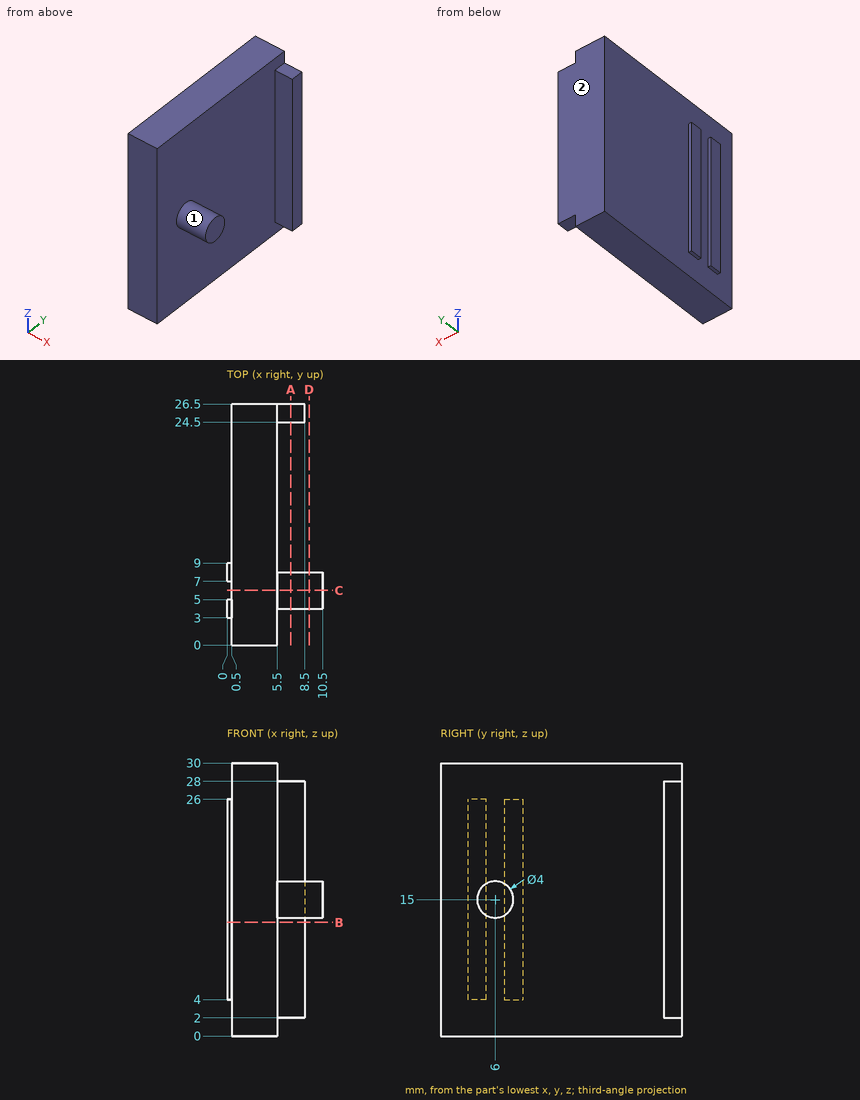
Geometry: see drawing. Coordinates: mm, zero at the bounding-box minimum. A direction names the side the tool comes from. Coordinates: 2 decimals unless noted, no trailing zeros. Loops run counter-clockwise (first coordinate to the right, second up) from the corner with the lowest first, then second, coordinate; pieces in that order, holes last. Notation, with made-up numbers: M -5,-26 L 12,-26 A18 ccw 12,-15 Z; hole C 73,-36 d8. An arc over 180 degrees is marked long. Put each result on its own line as item: value. Start each with the question number.
1) Contact query for flat-ended pins moving along their axis: pin 1 Ø3 at (y, z) = (6, 8) entering from +X; pin 2 Ø8 at (y, z) = (14.5, 12.5) entering from -X; pin 3 Ø0.6 at (y, z) = (25.5, 15) entering from +X. Output: stop coordinate, or through.
2) Cut plane D-D on x = 9. Return the cut outline in (y, z), then the cut area to 3 significant figures.
3) Ray query, L1, parallel to X at y = 20, z = 19.75; L2, parallel to X at y = 7.25, z = 8; L3, parallel to Y at x = 7.25, z = 8.5. Return the intervals inside material, ascending. Write a range as from..to.
4) Cut plane A-A on x = 7. Return the cut outline in (y, z), then the cut area to 3 significant figures.
5) Reachability of the marked faces 1 and 2 from +Z, -Z, +X, -X, +Y, -Y: full face, straight path, thin tool, end or side. Return the list, or none.
6) Cut plane B-B on z = 12.5. Return the cut outline in (x, y), then the cut area to 4 significant figures.
7) Cut plane C-C on y = 6. Return the cut outline in (x, z), then the cut area to 3 significant figures.
The answers:
1. pin 1: stops at x = 5.5
1. pin 2: stops at x = 0.5
1. pin 3: stops at x = 8.5
2. outline: C 6,15 d4
2. area: 12.6 mm²
3. L1: x = 0.5..5.5
3. L2: x = 0..5.5
3. L3: y = 24.5..26.5
4. outline: C 6,15 d4; M 24.5,2 L 26.5,2 L 26.5,28 L 24.5,28 Z
4. area: 64.6 mm²
5. face 1: +X
5. face 2: +Z, -Z, +X, -X, +Y
6. outline: M 0,3 L 0.5,3 L 0.5,0 L 5.5,0 L 5.5,24.5 L 8.5,24.5 L 8.5,26.5 L 0.5,26.5 L 0.5,9 L 0,9 L 0,7 L 0.5,7 L 0.5,5 L 0,5 Z
6. area: 140.5 mm²
7. outline: M 0.5,0 L 5.5,0 L 5.5,13 L 10.5,13 L 10.5,17 L 5.5,17 L 5.5,30 L 0.5,30 Z
7. area: 170 mm²
